from build123d import *

# Parameters (mm, degrees)
SKETCH1_W           = 23.368
SKETCH1_H           = 72.136
BOSS_EXTRUDE1_DEPTH = 2.54
SKETCH2_W           = 2.54
SKETCH2_H           = 58.42
CUT_EXTRUDE1_DEPTH  = 2.54
SKETCH3_W           = 2.54
SKETCH3_H           = 6.858
BOSS_EXTRUDE2_DEPTH = 8.128
SKETCH4_W           = 31.75
SKETCH4_H           = 58.42
BOSS_EXTRUDE3_DEPTH = 2.54
SKETCH5_W           = 2.54
SKETCH5_H           = 6.858
BOSS_EXTRUDE4_DEPTH = 2.54
BOSS_EXTRUDE5_START = -11.684
BOSS_EXTRUDE5_DEPTH = 52.578
BOSS_EXTRUDE6_DEPTH = 29.21
SKETCH10_W          = 7.62
SKETCH10_H          = 7.112
CUT_EXTRUDE2_DEPTH  = 31.242
SKETCH12_R          = 1.397
CUT_EXTRUDE3_DEPTH  = 21.3200001
BOSS_EXTRUDE7_DEPTH = 72.136
SKETCH14_W          = 8.128
SKETCH14_H          = 7.62
SKETCH14_W_2        = 11.43
SKETCH14_H_2        = 14.478
CUT_EXTRUDE4_DEPTH  = 31.242


with BuildPart() as part:
    # Sketch1 → Boss-Extrude1 (new body)
    with BuildSketch(Plane(origin=(0, 0, 0), x_dir=(1, 0, 0), z_dir=(0, 1, 0))):
        Rectangle(SKETCH1_W, SKETCH1_H)
    extrude(amount=BOSS_EXTRUDE1_DEPTH)

    # Sketch2 → Cut-Extrude1 (cut)
    with BuildSketch(Plane(origin=(0, 2.54, 0), x_dir=(1, 0, 0), z_dir=(0, 1, 0))):
        with Locations((10.414, 0)):
            Rectangle(SKETCH2_W, SKETCH2_H)
    extrude(amount=-CUT_EXTRUDE1_DEPTH, mode=Mode.SUBTRACT)

    # Sketch3 → Boss-Extrude2 (add)
    with BuildSketch(Plane(origin=(0, 2.54, 0), x_dir=(1, 0, 0), z_dir=(0, 1, 0))):
        with Locations((10.414, -32.639)):
            Rectangle(SKETCH3_W, SKETCH3_H)
        with Locations((10.414, 32.639)):
            Rectangle(SKETCH3_W, SKETCH3_H)
    extrude(amount=BOSS_EXTRUDE2_DEPTH)



with BuildPart() as body_2:
    # Sketch4 → Boss-Extrude3 (new body)
    with BuildSketch(Plane(origin=(0, 10.668, 0), x_dir=(1, 0, 0), z_dir=(0, 1, 0))):
        with Locations((25.019, 0)):
            Rectangle(SKETCH4_W, SKETCH4_H)
    extrude(amount=BOSS_EXTRUDE3_DEPTH)


with BuildPart() as part_1:
    add(part.part)

    add(body_2.part)  # Boss-Extrude4 merges body 2
    # Sketch5 → Boss-Extrude4 (add)
    with BuildSketch(Plane(origin=(0, 10.668, 0), x_dir=(1, 0, 0), z_dir=(0, 1, 0))):
        with Locations((10.414, -32.639)):
            Rectangle(SKETCH5_W, SKETCH5_H)
        with Locations((10.414, 32.639)):
            Rectangle(SKETCH5_W, SKETCH5_H)
    extrude(amount=BOSS_EXTRUDE4_DEPTH)

    # Sketch6 → Boss-Extrude5 (add)
    with BuildSketch(Plane(origin=(0, 0, 0), x_dir=(0, 0, -1), z_dir=(1, 0, 0)).offset(BOSS_EXTRUDE5_START)):
        with BuildLine():
            add(Edge.make_bspline(
                [(43.688, -7.112), (41.104515695, 2.079413445), (36.068, 2.54)],
                knots=[0, 0, 0, 0.627076912, 0.627076912, 0.627076912], degree=2))
            Line((36.068, 2.54), (36.068, -7.112))
            Line((36.068, -7.112), (43.688, -7.112))
        make_face()
    boss_extrude5 = extrude(amount=BOSS_EXTRUDE5_DEPTH)

    # Sketch7 → Boss-Extrude6 (add)
    with BuildSketch(Plane(origin=(11.684, 0, 0), x_dir=(0, 0, -1), z_dir=(1, 0, 0))):
        with BuildLine():
            add(Edge.make_bspline(
                [(36.068, 7.434839088), (33.013673055, 11.048422605), (29.21, 13.208)],
                knots=[0.279115305, 0.279115305, 0.279115305, 0.460674554, 0.460674554, 0.460674554], degree=2))
            Line((29.21, 13.208), (29.21, 10.668))
            Line((29.21, 10.668), (29.21, 0))
            Line((29.21, 0), (36.068, 0))
            Line((36.068, 0), (36.068, 2.54))
            Line((36.068, 2.54), (36.068, 7.434839088))
        make_face()
        with BuildLine():
            add(Edge.make_bspline(
                [(43.688, -7.112), (40.763488669, 1.879592133), (36.068, 7.434839088)],
                knots=[0, 0, 0, 0.279115305, 0.279115305, 0.279115305], degree=2))
            Line((36.068, 7.434839088), (36.068, 2.54))
            Line((36.068, 2.54), (36.068, 0))
            Line((36.068, 0), (29.21, 0))
            Line((29.21, 0), (29.21, -7.112))
            Line((29.21, -7.112), (43.688, -7.112))
        make_face()
    boss_extrude6 = extrude(amount=BOSS_EXTRUDE6_DEPTH)

    # Sketch10 → Cut-Extrude2 (cut)
    with BuildSketch(Plane(origin=(0, 25.4, 0), x_dir=(1, 0, 0), z_dir=(0, 1, 0))):
        with Locations((-7.874, 40.132)):
            Rectangle(SKETCH10_W, SKETCH10_H)
        with Locations((37.084, 40.132)):
            Rectangle(SKETCH10_W, SKETCH10_H)
    cut_extrude2 = extrude(amount=-CUT_EXTRUDE2_DEPTH, mode=Mode.SUBTRACT)

    # Sketch12 → Cut-Extrude3 (cut, through all)
    with BuildSketch(Plane.XZ.offset(7.112)):
        with Locations((-7.366, -38.608)):
            Circle(SKETCH12_R)
        with Locations((38.354, -38.608)):
            Circle(SKETCH12_R)
    cut_extrude3 = extrude(amount=-CUT_EXTRUDE3_DEPTH, mode=Mode.SUBTRACT)

    # Mirror1: Boss-Extrude5, Boss-Extrude6, Cut-Extrude2, Cut-Extrude3 across plane
    add(boss_extrude5.mirror(Plane.XY))
    add(boss_extrude6.mirror(Plane.XY))
    add(cut_extrude2.mirror(Plane.XY), mode=Mode.SUBTRACT)
    add(cut_extrude3.mirror(Plane.XY), mode=Mode.SUBTRACT)

    # Sketch13 → Boss-Extrude7 (add)
    with BuildSketch(Plane.XY.offset(36.068)):
        with BuildLine():
            Line((9.144, 2.54), (9.144, 13.208))
            add(Edge.make_bspline(
                [(-11.684, 2.54), (-2.430581771, 12.68572622), (9.144, 13.208)],
                knots=[0, 0, 0, 0.902085906, 0.902085906, 0.902085906], degree=2))
            Line((-11.684, 2.54), (9.144, 2.54))
        make_face()
    extrude(amount=-BOSS_EXTRUDE7_DEPTH)

    # Sketch14 → Cut-Extrude4 (cut)
    with BuildSketch(Plane(origin=(0, 25.4, 0), x_dir=(1, 0, 0), z_dir=(0, 1, 0))):
        with Locations((5.08, 39.878)):
            Rectangle(SKETCH14_W, SKETCH14_H)
        with Locations((17.289418024, -36.449)):
            Rectangle(SKETCH14_W_2, SKETCH14_H_2)
    extrude(amount=-CUT_EXTRUDE4_DEPTH, mode=Mode.SUBTRACT)


solid = part_1.part
Model file for the job. Use its own axes, mm. A direction names the side the tool comes from. Give positions to 0.01 mm unless a question says otherwise; leave off trailing zeros. Put each result on its own line as item: value. Start each with the question number.
(1) Pull direction Z, two halves, no side cores. Call faces 1 (the face through (9.144, 5, 0)), 2 (the face through (-8, -5.842, 41)), 3 (the face through (11.684, -4, -33)), 4 (the face through (2, 7, 36.068)): released by +Z, released by -Z, zero draft, split by the parting line, or undercut.
(2) Pin check, flat tips, straight feed: pin 1 Ø1 at (x, y) = (24, 6.5) entering from -Z; pin 2 Ø5.5 at (y, z) = (4.5, -11) entering from +X; pin 3 Ø6 at (x, y) = (-9, -2) entering from -Z. Stop position of each tip, or through.
(3) Tool access for faces 5 (the face through (17, -5.842, 36)), 6 (the face through (37, 1, -36.576)), 7 (the face through (-8, -2, -36.576)), 8 (the face through (5, -5.842, -40)): list every direction of +Z, -Z, +X, -X, +Y, -Y with a clear straight run to the whole face (end or side of a thin tool).
(4) Drill centre lines: L1, parallel to Z at x = 36, y = -5; L2, parallel to Y at x = 33, z = -13; L3, parallel to X at y = 2.5, z = 38.5. Where is each one in solid material? Low to high. Write a range as [from, to].
Results below:
1. face 1: undercut
1. face 2: zero draft
1. face 3: undercut
1. face 4: released by +Z
2. pin 1: stops at z = -37.21
2. pin 2: stops at x = 9.14
2. pin 3: stops at z = -36.58
3. face 5: +Z, +Y
3. face 6: -Z, +X, +Y
3. face 7: -Z, -X, +Y
3. face 8: -Z, +Y
4. L1: z = [-36.58, -29.21], [29.21, 36.58]
4. L2: y = [10.67, 13.21]
4. L3: x = [23, 33.27]
